from build123d import *

# Parameters (mm, degrees)
SKETCH9_R           = 30
SKETCH9_R_2         = 15
BOSS_EXTRUDE4_DEPTH = 25
BOSS_EXTRUDE5_DEPTH = 5
CUT_EXTRUDE2_DEPTH  = 99
SKETCH12_R          = 6
BOSS_EXTRUDE6_DEPTH = 9


with BuildPart() as part:
    # Sketch9 → Boss-Extrude4 (new body, symmetric)
    with BuildSketch(Plane(origin=(0, 0, 0), x_dir=(1, 0, 0), z_dir=(0, 1, 0))):
        Circle(SKETCH9_R)
        Circle(SKETCH9_R_2, mode=Mode.SUBTRACT)
    extrude(amount=BOSS_EXTRUDE4_DEPTH, both=True)

    # Sketch10 → Boss-Extrude5 (add, symmetric)
    with BuildSketch(Plane(origin=(0, 0, 0), x_dir=(1, 0, 0), z_dir=(0, 1, 0))):
        Polygon((29.859037173, -2.904806205), (17.655167851, -125.404806205), (-12.344832149, -125.404806205), (-29.859037173, -2.904806205), align=None)
    extrude(amount=BOSS_EXTRUDE5_DEPTH, both=True)

    # Sketch11 → Cut-Extrude2 (cut)
    with BuildSketch(Plane(origin=(0, 5, 0), x_dir=(1, 0, 0), z_dir=(0, 1, 0))):
        with BuildLine():
            Line((-14.716049093, -2.904806205), (14.716049093, -2.904806205))
            ThreePointArc((14.716049093, -2.904806205), (0, -15), (-14.716049093, -2.904806205))
        make_face()
    extrude(amount=-CUT_EXTRUDE2_DEPTH, mode=Mode.SUBTRACT)

    # Sketch12 → Boss-Extrude6 (add)
    with BuildSketch(Plane(origin=(29.852146538, 0, 2.973973023), x_dir=(0.0991327, 0, -0.995074222), z_dir=(0.995074222, 0, 0.0991327))):
        with BuildLine():
            Line((-123.036885537, 20), (-123.036885537, 5))
            Line((-123.036885537, 5), (-98.036885537, 5))
            Line((-98.036885537, 5), (-98.036885537, 20))
            ThreePointArc((-98.036885537, 20), (-110.536885537, 32.5), (-123.036885537, 20))
        make_face()
        with Locations((-110.536885537, 20)):
            Circle(SKETCH12_R, mode=Mode.SUBTRACT)
    extrude(amount=-BOSS_EXTRUDE6_DEPTH)


solid = part.part
The listing builds one solid part. Answer for the finished solid, in the listing's coordinates (mm). A direction names the side the tool comes from. Give positions to 0.01 mm unless a question says otherwise; leave off trailing zeros. Write each loop counter-clockwise with the first axis right and the second up, starting at its lowest first coordinate (ties: lowest second). Pieces come first, ordered by that corner, then holes. Notation, with made-up numbers: (80.25, 10) - (133.25, 10) arc R17 cw to (133.25, 36) - close; hole circle Ø6 at (84, 4). An arc over 180 degrees is marked (long way). One line per question, with ' | ' between items. Start each with the question number.
1. Section D-D, the plane y = 2 is taken. Determine the outline of the cut face in (x, z), then the cut area to 3 significant figures.
2. Section A-A, the plane z = 0 is taken. Determine the outline of the cut face in (x, y).
3. Determine the mould class of faces 5 (the face through (6, -25, -14)), 6 (the face through (9.92, 12.83, 112.25)), 7 (the face through (13.24, 12.605, 124.965)), 8 (the face through (15.05, 21.8, 106.83)) for opening direction Z: +Z half, -Z half, draft (parallel to the pull), parting line (faces both ways), or undercut.
4. Section B-B, the plane y = 23 is taken. Determine the outline of the cut face in (x, z).
5. Straight lines are drawn through the part: line 1 (Z direction, x = 0, y = 14); line 2 (Z direction, x = 0, y = -3.5). For each, find the intervals that lie inside material, in ascending order.
6. Given P1, Ø4, axis at y = -9, z = 3, coming from the +X side; P2, Ø4, axis at x = -7, y = -2, coming from the -Z side; P3, Ø18, axis at x = 0, z = 0, coming from the +Y side; P4, Ø2, axis at y = -5, z = 6.5, coming from the -X side, each flat-ended and moving along its own axis, determine where each tip first touches the part or whether it passes through.
7. For faces 1 (the face through (-20.79, 0.07, 66.33)), 2 (the face through (15.72, 12.4, 100.09)), 3 (the face through (-3.905, 0.35, -29.745)), 4 (the face through (6, 25, -14)), determine the directions among +Z, -Z, +X, -X, +Y, -Y from which every point of the face is accessible in a straight line to the end or side of a thin tool.
8. Section C-C, the plane x = 0 is taken. Determine the outline of the cut face in (y, z).
Result:
1) outline: (-29.48, 5.58) arc R30 ccw (long way) to (29.85, 3.04) - (17.66, 125.4) - (-12.34, 125.4) - close; hole circle Ø30 at (0, 0) | area: 6,380 mm2
2) outline: (-30, -25) - (-15, -25) - (-15, 25) - (-30, 25) - close; (15, -25) - (30, -25) - (30, 25) - (15, 25) - close
3) face 5: draft | face 6: undercut | face 7: +Z half | face 8: undercut
4) outline: circle Ø60 at (0, 0); (8.74, 124.15) - (9.42, 117.24) - (18.38, 118.14) - (17.69, 125.04) - close; (10.45, 106.9) - (11.14, 100) - (20.1, 100.89) - (19.41, 107.8) - close; hole circle Ø30 at (0, 0)
5) line 1: z = -30 to -15, 15 to 30 | line 2: z = -30 to -15, 15 to 125.4
6) P1: stops at x = 29.98 | P2: stops at z = -29.58 | P3: passes through | P4: stops at x = -29.49
7) face 1: +Z, -X, +Y, -Y | face 2: +X, +Y | face 3: none | face 4: -Z, +X, -X, +Y
8) outline: (-25, -30) - (25, -30) - (25, -15) - (-25, -15) - close; (-25, 15) - (25, 15) - (25, 30) - (5, 30) - (5, 125.4) - (-5, 125.4) - (-5, 30) - (-25, 30) - close
